Source: three-view drawing plus pictorial views. Frame: mm from the lowest corner of the part. Round coordinates to 2 decimals unless told otherwise and drop trailing zeros. Order: outer loops, then holes, each group sorted by start corner. A loop starts at its lowest first (then second) coordinate and runs counter-clockwise, first axis right, second up. Notation, with made-up numbers: M -28.75,-13 L 17.25,-13 A18 cw 17.25,14 Z; hole C 25,65 d9. An arc over 180 degrees is marked long. Return JSON: item names as keys, results as strings. Group by question number.
Q1. Mould query, pull axis X, two halves, no side actions, for the marked faces 1, 2 and 3. Classes: released by +X, released by -X, zero draft, split by the parting line, or undercut.
Q2. Cut plane D-D on x = 3.25. Output: boundary loops of the cut face in (y, z).
Q3. Ray query, probe 1 along Y at (x, z) = (11, 1.95); probe 2 along Y at (x, z) = (13.25, 1.5); probe 3 along X at (y, z) = (10, 0.7). Return the intervals inside material, ascending.
Q4. Contact query for flat-ended pins moving along their axis: pin 1 (1.5 mm diameter, centred on x = 16.5, z = 1, fed in from +Y); pin 2 (1 mm diameter, centred on x = 14.5, z = 2, fed in from -Y). Output: stop coordinate, or through.
Q5. Cut plane C-C on x = 20.5. Output: boundary loops of the cut face in (y, z).
Q6. Cut plane B-B on x = 11. Output: boundary loops of the cut face in (y, z), and give its area (3 significant figures).
Q7. Cut plane A-A on z = 2.35. Output: boundary loops of the cut face in (x, y), and give its area (3 significant figures).
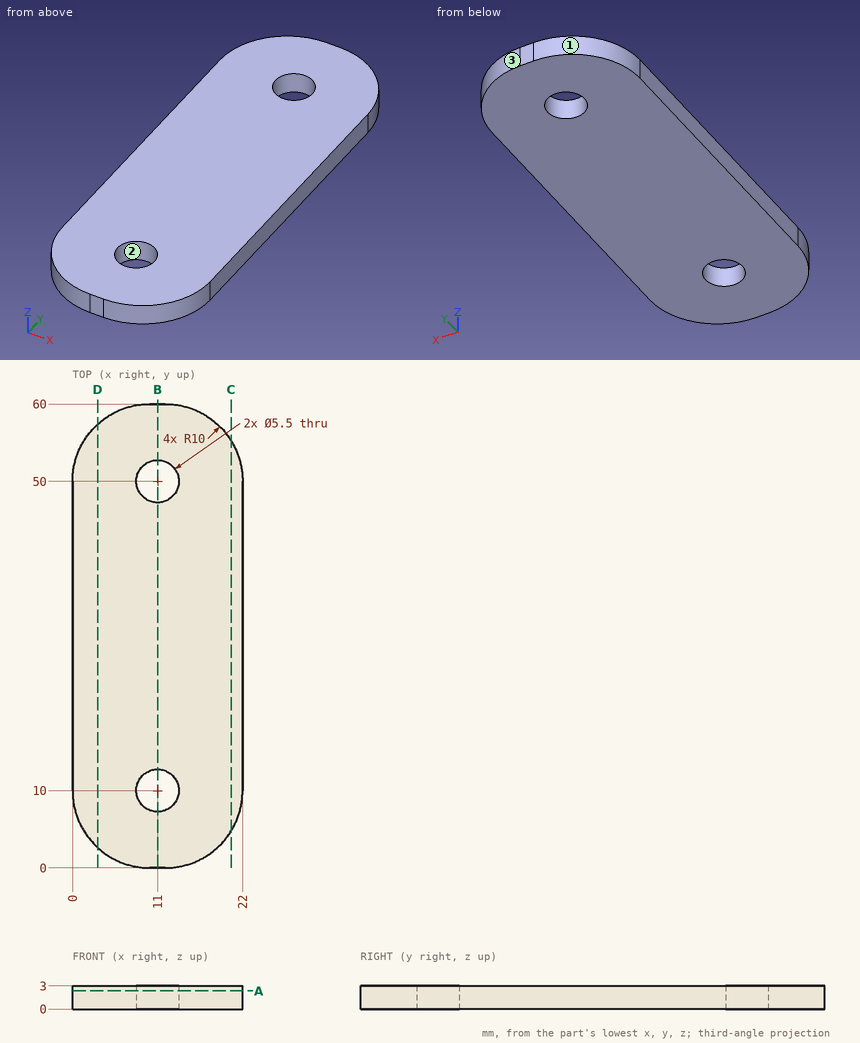
Result sheet:
{
 "1": {"face 1": "released by -X", "face 2": "undercut", "face 3": "released by +X"},
 "2": {"outline": "M 2.62,0 L 57.38,0 L 57.38,3 L 2.62,3 Z"},
 "3": {"probe 1": "y = 0 to 7.25, 12.75 to 47.25, 52.75 to 60", "probe 2": "y = 0.08 to 8.42, 11.58 to 48.42, 51.58 to 59.92", "probe 3": "x = 0 to 8.25, 13.75 to 22"},
 "4": {"pin 1": "stops at y = 59.27", "pin 2": "stops at y = 0.2"},
 "5": {"outline": "M 4.73,0 L 55.27,0 L 55.27,3 L 4.73,3 Z"},
 "6": {"outline": "M 0,0 L 7.25,0 L 7.25,3 L 0,3 Z; M 12.75,0 L 47.25,0 L 47.25,3 L 12.75,3 Z; M 52.75,0 L 60,0 L 60,3 L 52.75,3 Z", "area": "147 mm²"},
 "7": {"outline": "M 0,10 A10 ccw 10,0 L 12,0 A10 ccw 22,10 L 22,50 A10 ccw 12,60 L 10,60 A10 ccw 0,50 Z; hole C 11,10 d5.5; hole C 11,50 d5.5", "area": "1,190 mm²"}
}
